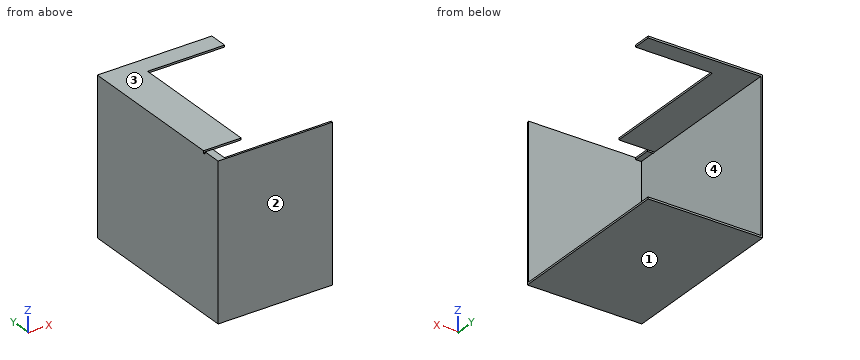
```python
from build123d import *

# Parameters (mm, degrees)
SKETCH_1_W          = 150
SKETCH_1_H          = 200
EXTRUDE_1_DEPTH     = 230
SHELL_1_T           = 2.5
CUT_EXTRUDE_1_DEPTH = 3
SKETCH_6_W          = 142.5
SKETCH_6_H          = 22.5
CUT_EXTRUDE_2_DEPTH = 30


with BuildPart() as part:
    # 草图1 → 凸台-拉伸1 (new body)
    with BuildSketch(Plane(origin=(0, 0, 0), x_dir=(1, 0, 0), z_dir=(0, 1, 0))):
        with Locations((75, -100)):
            Rectangle(SKETCH_1_W, SKETCH_1_H)
    extrude(amount=EXTRUDE_1_DEPTH)

    # 抽壳1
    shell_1_openings = [part.faces().sort_by_distance(p)[0] for p in [
        (150, 115, 100),
        (75, 230, 100),
    ]]
    offset(amount=SHELL_1_T, openings=shell_1_openings, kind=Kind.INTERSECTION)

    # 草图2 → 切除-拉伸1 (cut)
    with BuildSketch(Plane.XY.offset(202.5)):
        Polygon((-2.5, 25.5), (47.5, 25.5), (47.5, 205.5), (150, 205.5), (150, 30.5), (150, 27.5), (150, 22.5), (-2.5, 22.5), align=None)
    extrude(amount=-CUT_EXTRUDE_1_DEPTH, mode=Mode.SUBTRACT)

    # 草图6 → 切除-拉伸2 (cut)
    with BuildSketch(Plane.XY.offset(202.5)):
        with Locations((78.75, 11.25)):
            Rectangle(SKETCH_6_W, SKETCH_6_H)
    extrude(amount=-CUT_EXTRUDE_2_DEPTH, mode=Mode.SUBTRACT)


solid = part.part
```
Geometry: final body of the model. Coordinates: model frame, mm. Face numbers are marked on the shaded views. A direction names the side the tool comes from. Round coordinates to 2 decimals unless told otherwise and drop trailing zeros. Order: outer loops, then holes, each group sorted by start corner. A loop starts at its lowest first (then second) coordinate and runs counter-clockwise, first axis right, second up. Notation, with made-up numbers: (11, -2) -> (41, -2) arc R15 cw to (41, 19) -> close; hole circle Ø10 at (-9, 19.5). An arc over 180 degrees is marked (long way). Write each question's results on one line, items separated by ' | '.
Q1. Pull-direction query (Y, two-part tool) for the marked faces 1 and 2; classes: released by +Y, released by -Y, zero draft, split by the parting line, or undercut.
Response values:
face 1: zero draft | face 2: released by -Y
Q2. Section query C-C (y = 181.5). Output: boundary loops of the cut face in (x, z).
Response values:
outline: (-2.5, -2.5) -> (150, -2.5) -> (150, 0) -> (0, 0) -> (0, 200) -> (47.5, 200) -> (47.5, 202.5) -> (-2.5, 202.5) -> close
Q3. Pin query (flat end, axial travel): pin 1 Ø6 at (x, y) = (73.5, 80.5) entering from +Z; pin 2 Ø0.8 at (y, z) = (122.5, 201.5) entering from +X; pin 3 Ø1.2 at (y, z) = (11.5, 201.5) entering from +X. Return the tip coordinate at first contact, or that it passes through.
Response values:
pin 1: z = 0 | pin 2: x = 47.5 | pin 3: x = 7.5
Q4. Section query B-B (z = 19). Output: boundary loops of the cut face in (x, y).
Response values:
outline: (-2.5, -2.5) -> (150, -2.5) -> (150, 0) -> (0, 0) -> (0, 230) -> (-2.5, 230) -> close
Q5. Access query for the marked faces 3 and 4. Directions: +Z, -Z, +X, -X, +Y, -Y. A direction counts if a zero-diameter tool reaches every point of the face in a straight line with its end or side. Return the directions, or none.
Response values:
face 3: +Z, +X, -X, +Y, -Y | face 4: +X, +Y
Q6. Section query A-A (x = 117). Output: boundary loops of the cut face in (y, z).
Response values:
outline: (-2.5, -2.5) -> (230, -2.5) -> (230, 0) -> (0, 0) -> (0, 202.5) -> (-2.5, 202.5) -> close; (205.5, 200) -> (230, 200) -> (230, 202.5) -> (205.5, 202.5) -> close
Q7. Ray query, line 1 along Z through (x, y) = (46.5, 27); line 2 along Y through (x, z) = (135, 21). Return the intervals inside material, ascending.
Response values:
line 1: -2.5 to 0, 200 to 202.5 | line 2: -2.5 to 0
